from build123d import *

# Parameters (mm, degrees)
BOSS_EXTRUDE1_DEPTH = 3
BOSS_EXTRUDE2_DEPTH = 4


with BuildPart() as part:
    # Sketch1 → Boss-Extrude1 (new body)
    with BuildSketch(Plane(origin=(0, 0, 0), x_dir=(1, 0, 0), z_dir=(0, 1, 0))):
        Polygon((0, 0), (-4, 4), (0, 4), align=None)
    extrude(amount=BOSS_EXTRUDE1_DEPTH)

    # Sketch2 → Boss-Extrude2 (add)
    with BuildSketch(Plane(origin=(0, 0, -4), x_dir=(-1, 0, 0), z_dir=(0, 0, -1))):
        Polygon((1.152291055, 5), (3.152291055, 3), (0, 3), (0, 0), (-4, 0), (-4, 5), align=None)
    extrude(amount=-BOSS_EXTRUDE2_DEPTH)


solid = part.part
Verification items for the finished model (mm, model axes). A direction names the side the tool comes from. Coordinates: 2 decimals unless noted, no trailing zeros. Loops run counter-clockwise (first coordinate to the right, second up) from the corner with the lowest first, then second, coordinate; pieces in that order, holes last. Notation, with made-up numbers: (28.5, 78) -> (68.5, 78) arc R6 cw to (68.5, 82) -> close; hole circle Ø2 at (47.5, -12.75). An arc over 180 degrees is marked (long way). Answer as a JSON object with one key per item and string values. Group by question number.
Item 1: Sectioned sample at D-D on y = 4.25. Record the boundary of the cut face in (x, z), plus the area to 3 significant figures.
Item 2: Depth check by flat-ended pin: pin 1 (2 mm diameter, centred on y = 1, z = -3.5, fed in from -X). Enter the tip coordinate at first touch or a pass-through.
Item 3: Sectioned sample at B-B on x = -0.25. Record the boundary of the cut face in (y, z), plus the area to 4 significant figures.
Item 4: Scan lines: probe 1 along Y at (x, z) = (-0.75, -0.5); probe 2 along X at (y, z) = (4.2, -0.35); probe 3 along Z at (x, y) = (-2.75, 1.9). Record each from-to range of solid material in increasing order.
Item 5: Sectioned sample at A-A on z = -2.3. Record the boundary of the cut face in (x, y), plus the area to 3 significant figures.
Item 6: Sectioned sample at C-C on y = 1.8. Record the boundary of the cut face in (x, z), plus the area to 3 significant figures.
Item 7: Tool access check on faces 1 (the flat face through (0, 3, -4)), 2 (the flat face through (-3.4, 3, -3.7)), 3 (the flat face through (-2, 3, -1)). Record the directions out of +Z, -Z, +X, -X, +Y, -Y that give a thin tool (end or side, any length) a straight path to the whole face; none if there is none.
Evaluation:
{
 "1": {"outline": "(-1.9, -4) -> (4, -4) -> (4, 0) -> (-1.9, 0) -> close", "area": "23.6 mm²"},
 "2": {"pin 1": "stops at x = -4"},
 "3": {"outline": "(0, -4) -> (5, -4) -> (5, 0) -> (3, 0) -> (3, -0.25) -> (0, -0.25) -> close", "area": "19.25 mm²"},
 "4": {"probe 1": "y = 3 to 5", "probe 2": "x = -1.95 to 4", "probe 3": "z = -4 to -2.75"},
 "5": {"outline": "(-3.15, 3) -> (-2.3, 3) -> (-2.3, 0) -> (4, 0) -> (4, 5) -> (-1.15, 5) -> close", "area": "31.2 mm²"},
 "6": {"outline": "(-4, -4) -> (4, -4) -> (4, 0) -> (0, 0) -> close", "area": "24.0 mm²"},
 "7": {"face 1": "-Z, +X, -X, +Y, -Y", "face 2": "+Z, -Z, -X, +Y", "face 3": "+Z, -X, -Y"}
}
